Part model, mm, in its own coordinate system. Face numbers are marked on the shaded views. A direction names the side the tool comes from. Give positions to 0.01 mm unless a question says otherwise; leave off trailing zeros. Write each loop counter-clockwise with the first axis right and the second up, starting at its lowest first coordinate (ties: lowest second). Pieces come first, ordered by that corner, then holes. Notation, with made-up numbers: M -1.5,70.5 L 10.5,70.5 A17 cw 10.5,85.5 Z; hole C -5,45 d1. An arc over 180 degrees is marked long. Use CSV: the item, a comma, the result in double quotes. Start each with the question number.
Item 1: Cut at B-B (z = 10.25). List the corners of the cut face in (x, y), then the cut area to 3 significant figures.
Item 2: Cut at A-A (z = 3.75). List the corners of the cut face in (x, y), then the cut area to 3 significant figures.
Item 3: Drill centre lines: line 1 (Z direction, x = 2.25, y = -3.25); line 2 (X direction, y = -2, z = 8.75); line 3 (Y direction, x = -0.25, z = 9.75). Where is each one in solid material? Low to high. Write a range as [from, to].
Item 4: Which spindle directions (+Z, -Z, +X, -X, +Y, -Y) get a long thin tool onto all of the face, cutting with end or side? Do the marked faces 1 and 2. Say none if no direction does.
Item 5: Pin check, flat tips, straight feed: pin 1 (2 mm diameter, centred on x = -7, y = -0.5, fed in from +Z); pin 2 (6 mm diameter, centred on y = -5.5, z = 8.5, fed in from -X); pin 3 (1 mm diameter, centred on y = 5.5, z = 14, fed in from -X). Stop position of each tip, or through.
from build123d import *

# Parameters (mm, degrees)
SKETCH_R     = 2.9
PAD_DEPTH    = 8
SKETCH001_R  = 9
PAD001_DEPTH = 10
FILLET_R     = 4
CHAMFER_SIZE = 1


with BuildPart() as part:
    # Sketch → Pad (new body)
    with BuildSketch(Plane.XY):
        Circle(SKETCH_R)
    extrude(amount=PAD_DEPTH)

    # Sketch001 (on Face3 of Pad) → Pad001 (join)
    with BuildSketch(Plane.XY.offset(8)):
        with Locations((-0.011619, 0.070584)):
            Circle(SKETCH001_R)
    extrude(amount=PAD001_DEPTH)

    # Fillet
    fillet_edges = [part.edges().sort_by_distance(p)[0] for p in [
        (-9.011619, 0.070584, 18),
    ]]
    fillet(fillet_edges, radius=FILLET_R)

    # Chamfer
    chamfer_edges = [part.edges().sort_by_distance(p)[0] for p in [
        (-2.9, 0, 0),
    ]]
    chamfer(chamfer_edges, length=CHAMFER_SIZE)


solid = part.part
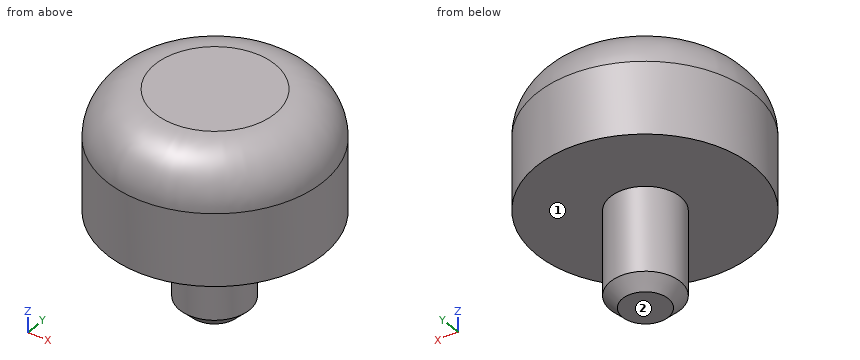
Worked answers:
1,outline,"C -0.01,0.07 d18"
1,area,"254 mm^2"
2,outline,"C 0,0 d5.8"
2,area,"26.4 mm^2"
3,line 1,"z = [8, 18]"
3,line 2,"x = [-8.77, 8.75]"
3,line 3,"y = [-8.93, 9.07]"
4,face 1,"-Z"
4,face 2,"-Z, +X, -X, +Y, -Y"
5,pin 1,"stops at z = 17.87"
5,pin 2,"stops at x = -8.64"
5,pin 3,"stops at x = -7.54"
